```python
from build123d import *

# Parameters (mm, degrees)
PCB_DEPTH                        = 1.6
SKETCH2_W                        = 38
SKETCH2_H                        = 5.5
J2_HEADER_AND_DUPONT_PLUGS_DEPTH = 20
SKETCH3_W                        = 2
SKETCH3_H                        = 8
TOF_CARRIER_LEFT_DEPTH           = 14
SKETCH4_W                        = 8
SKETCH4_H                        = 2
TOF_CARRIER_AHEAD_DEPTH          = 14
SKETCH5_W                        = 2
SKETCH5_H                        = 8
TOF_CARRIER_RIGHT_DEPTH          = 14


with BuildPart() as part:
    # Sketch1 → PCB (new body)
    with BuildSketch(Plane(origin=(0, -1.6, 0), x_dir=(1, 0, 0), z_dir=(0, 1, 0))):
        Polygon((-43, 0), (43, 0), (43, 22), (20.5, 41.843134833), (-20.5, 41.843134833), (-43, 22), align=None)
    extrude(amount=PCB_DEPTH)

    # Sketch2 → J2 Header And Dupont Plugs (add)
    with BuildSketch(Plane(origin=(0, -20, 0), x_dir=(1, 0, 0), z_dir=(0, 1, 0))):
        with Locations((0, 3.55)):
            Rectangle(SKETCH2_W, SKETCH2_H)
    extrude(amount=J2_HEADER_AND_DUPONT_PLUGS_DEPTH)

    # Sketch3 → ToF Carrier Left (add)
    with BuildSketch(Plane(origin=(0, 0, 0), x_dir=(1, 0, 0), z_dir=(0, 1, 0))):
        with Locations((-23.5, 32)):
            Rectangle(SKETCH3_W, SKETCH3_H)
    extrude(amount=TOF_CARRIER_LEFT_DEPTH)

    # Sketch4 → ToF Carrier Ahead (add)
    with BuildSketch(Plane(origin=(0, 0, 0), x_dir=(1, 0, 0), z_dir=(0, 1, 0))):
        with Locations((0, 42)):
            Rectangle(SKETCH4_W, SKETCH4_H)
    extrude(amount=TOF_CARRIER_AHEAD_DEPTH)

    # Sketch5 → ToF Carrier Right (add)
    with BuildSketch(Plane(origin=(0, 0, 0), x_dir=(1, 0, 0), z_dir=(0, 1, 0))):
        with Locations((23.5, 32)):
            Rectangle(SKETCH5_W, SKETCH5_H)
    extrude(amount=TOF_CARRIER_RIGHT_DEPTH)


solid = part.part
```
Here's how the part is built. I have some questions about the finished solid (model axes, mm). A direction names the side the tool comes from. Give positions to 0.01 mm unless a question says otherwise; leave off trailing zeros. Order: outer loops, then holes, each group sorted by start corner. A loop starts at its lowest first (then second) coordinate and runs counter-clockwise, first axis right, second up. Notation, with made-up numbers: M -27.5,66.25 L -13.5,66.25 A17 ccw -13.5,72.25 Z; hole C 80,-31.75 d3. An arc over 180 degrees is marked long. Use a Markdown table: item, result. Add a question column.
1. For pin 1 Ø6 at (y, z) = (-14.5, -5) entering from -X; pin 2 Ø9 at (y, z) = (5.5, -33.5) entering from +X; pin 3 Ø4 at (y, z) = (9.5, -30.5) entering from -X; pin 4 Ø1.5 at (x, y) = (-21.5, 9.5) entering from +Z, each with a flat end and sliding along its axis, tell me the tip position at first contact or that it passes through.
2. Suppose I cut it at A-A (y = 5). List the corners of the cut face in (x, z) for me.
3. On a 3-axis mill with a long thin cutter (end or side, diameter ignored), from which of +Z, -Z, +X, -X, +Y, -Y can I reach the whole of each face in a straight line? I mean faces 5 (the flat face through (0, -11, -0.8)), 6 (the flat face through (22.5, 7, -32)), 7 (the flat face through (0, 7, -41)), 8 (the flat face through (-24, 7, -36)), 9 (the flat face through (-4, 7, -42)). Say none if no direction works.
4. I need wall thicknesses on probe 1 along Y at (x, z) = (28.5, -13.5); probe 2 along Z at (x, y) = (2, -10); probe 3 along Z at (x, y) = (-24, 9). Which ranges of each line are inside material? Lowest first, please. Write a range as from..to.
5. Suppose I cut it at C-C (z = -14.5). List the corners of the cut face in (x, y) for me, and give its area (3 significant figures).
6. Suppose I cut it at B-B (x = -10). List the corners of the cut face in (y, z) for me.
7. Suppose I cut it at D-D (x = 0). List the corners of the cut face in (y, z) for me.
8. If we mould it in two halves opening along X, with no side actions, what happens to faces 1 (the flat face through (-19, -11, -4)), 2 (the flat face through (-1, 0, -21)), 3 (the flat face through (-24, 7, -28)), 4 (the flat face through (43, -1, -11))? For each: +X half, -X half, draft (parallel to the pull), parting line (faces both ways), or undercut.
Results list:
| question | item | result |
|---|---|---|
| 1 | pin 1 | stops at x = -19 |
| 1 | pin 2 | stops at x = 24.5 |
| 1 | pin 3 | stops at x = -24.5 |
| 1 | pin 4 | passes through |
| 2 | outline | M -24.5,-36 L -22.5,-36 L -22.5,-28 L -24.5,-28 Z; M -4,-43 L 4,-43 L 4,-41 L -4,-41 Z; M 22.5,-36 L 24.5,-36 L 24.5,-28 L 22.5,-28 Z |
| 3 | face 5 | +Z, +X, -X, -Y |
| 3 | face 6 | +Z, -Z, +Y |
| 3 | face 7 | +Z, +X, -X, +Y |
| 3 | face 8 | -Z, +X, -X, +Y |
| 3 | face 9 | +Z, -Z, -X, +Y |
| 4 | probe 1 | y = -1.6..0 |
| 4 | probe 2 | z = -6.3..-0.8 |
| 4 | probe 3 | z = -36..-28 |
| 5 | outline | M -43,-1.6 L 43,-1.6 L 43,0 L -43,0 Z |
| 5 | area | 138 mm² |
| 6 | outline | M -20,-6.3 L -1.6,-6.3 L -1.6,-41.84 L 0,-41.84 L 0,0 L -1.6,0 L -1.6,-0.8 L -20,-0.8 Z |
| 7 | outline | M -20,-6.3 L -1.6,-6.3 L -1.6,-41.84 L 0,-41.84 L 0,-43 L 14,-43 L 14,-41 L 0,-41 L 0,0 L -1.6,0 L -1.6,-0.8 L -20,-0.8 Z |
| 8 | face 1 | -X half |
| 8 | face 2 | undercut |
| 8 | face 3 | draft |
| 8 | face 4 | +X half |
